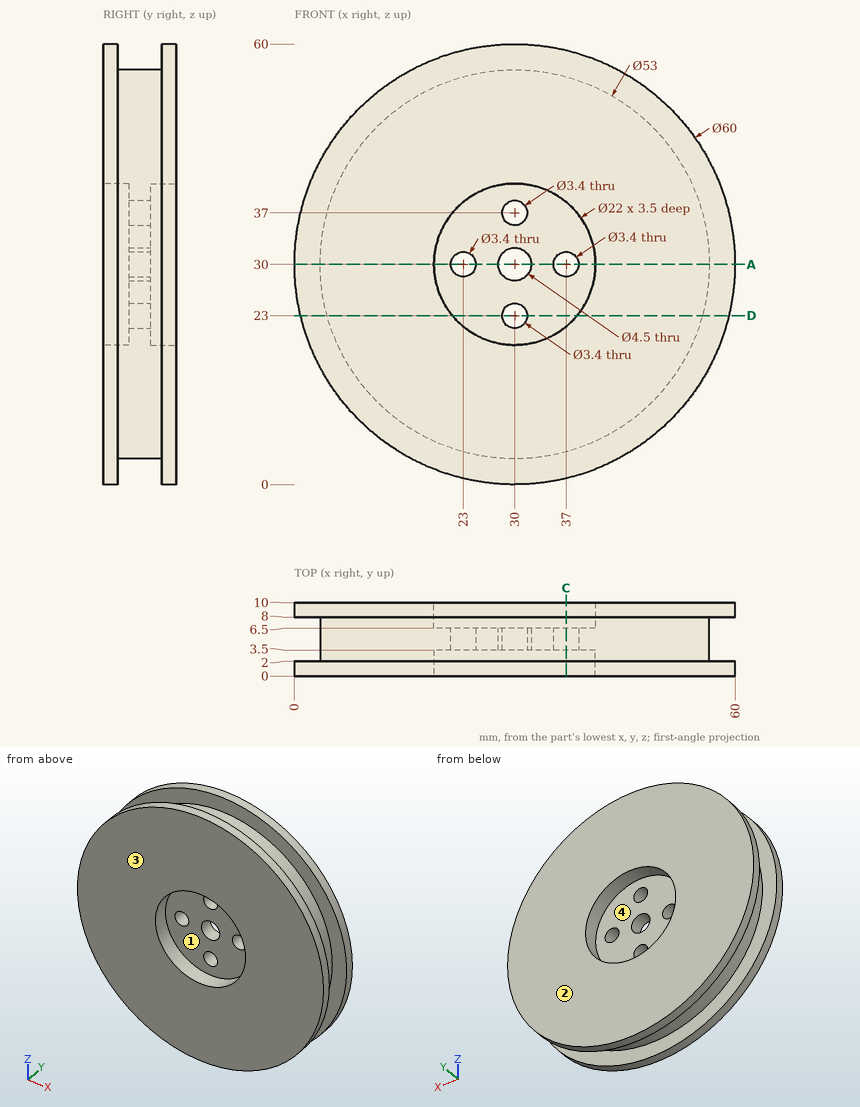
Geometry: see drawing. Coordinates: mm, zero at the bounding-box minimum. A direction names the side the tool comes from. Coordinates: 2 decimals unless noted, no trailing zeros. Loops run counter-clockwise (first coordinate to the right, second up) from the corner with the lowest first, then second, coordinate; pieces in that order, holes last.
Q1. Set-up query: the marked faces 3 and 4. Return all of +Z, -Z, +X, -X, +Y, -Y with unobstructed straight access to the full face (end or side cutting, diameter ignored); none if empty.
Q2. Material intervals for line 1 (Z direction, x = 30, y = 4.85); line 2 (Y direction, x = 55, z = 20), sorted ascending.
Q3. Cut plane A-A (z = 30). Give the number of separate pieces and of enclosed holes in the cut face, then the cut area to 3 significant figures.
Q4. Cut plane C-C (x = 37). Output: boundary loops of the cut face in (y, z).
Q5. Cut plane D-D (z = 23). Output: boundary loops of the cut face in (x, y).
Q6. Draft query along Z for the marked faces 1 and 2. Return one class per face: +Z half, -Z half, draft (parallel to the pull), parting line (faces both ways), or undercut.
Q7. Contact query for flat-ended pins moving along their axis: pin 1 (3 mm diameter, centred on y = 5.5, z = 16.5, fed in from -X); pin 2 (1.5 mm diameter, centred on x = 22.5, y = 6.5, fed in from +Z); pin 3 (5 mm diameter, centred on x = 33.5, z = 24.5, fed in from -Y). Output: stop coordinate, or through.
Working result:
1. face 3: +Z, -Z, +X, -X, -Y
1. face 4: +Y
2. line 1: z = 3.5 to 21.3, 24.7 to 27.75, 32.25 to 35.3, 38.7 to 56.5
2. line 2: y = 0 to 2, 8 to 10
3. separate pieces: 4
3. enclosed holes: 0
3. area: 370 mm2
4. outline: (0, 0.83) - (2, 0.83) - (2, 4.44) - (8, 4.44) - (8, 0.83) - (10, 0.83) - (10, 21.51) - (6.5, 21.51) - (6.5, 28.3) - (3.5, 28.3) - (3.5, 21.51) - (0, 21.51) - close; (0, 38.49) - (3.5, 38.49) - (3.5, 31.7) - (6.5, 31.7) - (6.5, 38.49) - (10, 38.49) - (10, 59.17) - (8, 59.17) - (8, 55.56) - (2, 55.56) - (2, 59.17) - (0, 59.17) - close
5. outline: (0.83, 0) - (21.51, 0) - (21.51, 3.5) - (28.3, 3.5) - (28.3, 6.5) - (21.51, 6.5) - (21.51, 10) - (0.83, 10) - (0.83, 8) - (4.44, 8) - (4.44, 2) - (0.83, 2) - close; (31.7, 3.5) - (38.49, 3.5) - (38.49, 0) - (59.17, 0) - (59.17, 2) - (55.56, 2) - (55.56, 8) - (59.17, 8) - (59.17, 10) - (38.49, 10) - (38.49, 6.5) - (31.7, 6.5) - close
6. face 1: undercut
6. face 2: draft
7. pin 1: stops at x = 6.37
7. pin 2: stops at z = 55.63
7. pin 3: stops at y = 3.5
